The model under review builds one solid part; all positions refer to its coordinate system, in mm. Face numbers are marked on the shaded views. A direction names the side the tool comes from. Coordinates: 2 decimals unless noted, no trailing zeros. Loops run counter-clockwise (first coordinate to the right, second up) from the corner with the lowest first, then second, coordinate; pieces in that order, holes last. Notation, with made-up numbers: M 0,38 L 44,38 A18 cw 44,67 Z; hole C 75,-8 d7. An arc over 180 degrees is marked long. Use one line per item in the form item = value.
```python
from build123d import *

# Parameters (mm, degrees)
SKETCH_2_R           = 38.25
SKETCH_2_R_2         = 1.3
EXTRUDE_1_DEPTH      = 27
EXTRUDE_2_DEPTH      = 6.2
SKETCH_4_R           = 19.25
CUT_EXTRUDE_1_DEPTH  = 1.7
SKETCH_5_R           = 14.9
CUT_EXTRUDE_2_DEPTH  = 3.2
SKETCH_6_R           = 1.5
CUT_EXTRUDE_3_DEPTH  = 8
SKETCH_7_R           = 2
CUT_EXTRUDE_4_DEPTH  = 4.5
SKETCH_8_R           = 32.3
EXTRUDE_3_DEPTH      = 39.3
FILLET_1_R           = 7
FILLET_2_R           = 10
SKETCH_9_W           = 22
SKETCH_9_H           = 6
CUT_EXTRUDE_5_DEPTH  = 15
SKETCH_10_W          = 22
SKETCH_10_H          = 13
CUT_EXTRUDE_6_DEPTH  = 15
SKETCH_12_R          = 9.8
CUT_EXTRUDE_7_DEPTH  = 6.5
SKETCH_13_R          = 4
CUT_EXTRUDE_8_DEPTH  = 6
SKETCH_14_R          = 2.7
CUT_EXTRUDE_9_DEPTH  = 7
SKETCH_15_R          = 1.2
CUT_EXTRUDE_10_DEPTH = 4
SKETCH_16_R          = 1.3
SKETCH_16_R_2        = 1.2
EXTRUDE_4_DEPTH      = 12
SKETCH_18_R          = 1.3
EXTRUDE_5_DEPTH      = 9
SKETCH_19_R          = 1.5
CUT_EXTRUDE_11_DEPTH = 10


with BuildPart() as part:
    # 草图2 → 凸台-拉伸1 (new body)
    with BuildSketch(Plane(origin=(0, 0, 0), x_dir=(1, 0, 0), z_dir=(0, 1, 0))):
        with Locations(Location((0, 0, 0), (0, 0, 270))):
            Circle(SKETCH_2_R)
        with Locations(Location((0, 34.5, 0), (0, 0, 270))):
            Circle(SKETCH_2_R_2, mode=Mode.SUBTRACT)
        with Locations(Location((-24.395183951, 24.395183951, 0), (0, 0, 270))):
            Circle(SKETCH_2_R_2, mode=Mode.SUBTRACT)
        with Locations(Location((-34.5, 0, 0), (0, 0, 270))):
            Circle(SKETCH_2_R_2, mode=Mode.SUBTRACT)
        with Locations(Location((-24.395183951, -24.395183951, 0), (0, 0, 270))):
            Circle(SKETCH_2_R_2, mode=Mode.SUBTRACT)
        with Locations(Location((0, -34.5, 0), (0, 0, 270))):
            Circle(SKETCH_2_R_2, mode=Mode.SUBTRACT)
        with Locations(Location((24.395183951, -24.395183951, 0), (0, 0, 270))):
            Circle(SKETCH_2_R_2, mode=Mode.SUBTRACT)
        with Locations(Location((34.5, 0, 0), (0, 0, 270))):
            Circle(SKETCH_2_R_2, mode=Mode.SUBTRACT)
        with Locations(Location((24.395183951, 24.395183951, 0), (0, 0, 270))):
            Circle(SKETCH_2_R_2, mode=Mode.SUBTRACT)
    extrude(amount=EXTRUDE_1_DEPTH)

    # 草图3 → 凸台-拉伸2 (add)
    with BuildSketch(Plane(origin=(0, 27, 0), x_dir=(1, 0, 0), z_dir=(0, 1, 0))):
        with BuildLine():
            Line((-13.978197309, 23.1), (13.978197309, 23.1))
            ThreePointArc((13.978197309, 23.1), (27, 0), (13.978197309, -23.1))
            Line((13.978197309, -23.1), (-13.978197309, -23.1))
            ThreePointArc((-13.978197309, -23.1), (-27, 0), (-13.978197309, 23.1))
        make_face()
    extrude(amount=EXTRUDE_2_DEPTH)

    # 草图4 → 切除-拉伸1 (cut)
    with BuildSketch(Plane(origin=(0, 33.2, 0), x_dir=(1, 0, 0), z_dir=(0, 1, 0))):
        with Locations(Location((0, 0, 0), (0, 0, 270))):
            Circle(SKETCH_4_R)
    extrude(amount=-CUT_EXTRUDE_1_DEPTH, mode=Mode.SUBTRACT)

    # 草图5 → 切除-拉伸2 (cut)
    with BuildSketch(Plane(origin=(0, 33.2, 0), x_dir=(1, 0, 0), z_dir=(0, 1, 0))):
        with Locations(Location((0, 0, 0), (0, 0, 270))):
            Circle(SKETCH_5_R)
    extrude(amount=-CUT_EXTRUDE_2_DEPTH, mode=Mode.SUBTRACT)

    # 草图6 → 切除-拉伸3 (cut)
    with BuildSketch(Plane(origin=(0, 30, 0), x_dir=(1, 0, 0), z_dir=(0, 1, 0))):
        with Locations(Location((0, -12.5, 0), (0, 0, 270))):
            Circle(SKETCH_6_R)
        with Locations(Location((10.825317547, -6.25, 0), (0, 0, 270))):
            Circle(SKETCH_6_R)
        with Locations(Location((10.825317547, 6.25, 0), (0, 0, 270))):
            Circle(SKETCH_6_R)
        with Locations(Location((-10.825317547, -6.25, 0), (0, 0, 270))):
            Circle(SKETCH_6_R)
        with Locations(Location((-10.825317547, 6.25, 0), (0, 0, 270))):
            Circle(SKETCH_6_R)
        with Locations(Location((0, 12.5, 0), (0, 0, 270))):
            Circle(SKETCH_6_R)
    extrude(amount=-CUT_EXTRUDE_3_DEPTH, mode=Mode.SUBTRACT)

    # 草图7 → 切除-拉伸4 (cut)
    with BuildSketch(Plane(origin=(0, 30, 0), x_dir=(1, 0, 0), z_dir=(0, 1, 0))):
        with Locations(Location((-12.5, 0, 0), (0, 0, 270))):
            Circle(SKETCH_7_R)
        with Locations(Location((6.25, -10.825317547, 0), (0, 0, 270))):
            Circle(SKETCH_7_R)
        with Locations(Location((6.25, 10.825317547, 0), (0, 0, 270))):
            Circle(SKETCH_7_R)
    extrude(amount=-CUT_EXTRUDE_4_DEPTH, mode=Mode.SUBTRACT)

    # 草图8 → 凸台-拉伸3 (add)
    with BuildSketch(Plane(origin=(0, 0, 0), x_dir=(1, 0, 0), z_dir=(0, 1, 0))):
        with Locations(Location((0, 0, 0), (0, 0, 270))):
            Circle(SKETCH_8_R)
    extrude(amount=-EXTRUDE_3_DEPTH)

    # 圆角1
    fillet_1_edges = [part.edges().sort_by_distance(p)[0] for p in [
        (0, -39.3, -32.3),
    ]]
    fillet(fillet_1_edges, radius=FILLET_1_R)

    # 圆角2
    fillet_2_edges = [part.edges().sort_by_distance(p)[0] for p in [
        (-13.978197309, 30.1, -23.1),
        (-13.978197309, 30.1, 23.1),
        (13.978197309, 30.1, 23.1),
        (13.978197309, 30.1, -23.1),
    ]]
    fillet(fillet_2_edges, radius=FILLET_2_R)

    # 草图9 → 切除-拉伸5 (cut)
    with BuildSketch(Plane.XY.offset(40)):
        with Locations((0, -29.3)):
            Rectangle(SKETCH_9_W, SKETCH_9_H)
    extrude(amount=-CUT_EXTRUDE_5_DEPTH, mode=Mode.SUBTRACT)

    # 草图10 → 切除-拉伸6 (cut)
    with BuildSketch(Plane.XY.offset(-40)):
        with Locations((0, -30.8)):
            Rectangle(SKETCH_10_W, SKETCH_10_H)
    extrude(amount=CUT_EXTRUDE_6_DEPTH, mode=Mode.SUBTRACT)

    # 草图12 → 切除-拉伸7 (cut)
    with BuildSketch(Plane(origin=(0, 30, 0), x_dir=(1, 0, 0), z_dir=(0, 1, 0))):
        with Locations(Location((0, 0, 0), (0, 0, 270))):
            Circle(SKETCH_12_R)
    extrude(amount=-CUT_EXTRUDE_7_DEPTH, mode=Mode.SUBTRACT)

    # 草图13 → 切除-拉伸8 (cut)
    with BuildSketch(Plane(origin=(0, 23.5, 0), x_dir=(1, 0, 0), z_dir=(0, 1, 0))):
        with Locations(Location((0, 0, 0), (0, 0, 270))):
            Circle(SKETCH_13_R)
    extrude(amount=-CUT_EXTRUDE_8_DEPTH, mode=Mode.SUBTRACT)

    # 草图14 → 切除-拉伸9 (cut)
    with BuildSketch(Plane(origin=(0, 27, 0), x_dir=(1, 0, 0), z_dir=(0, 1, 0))):
        with Locations(Location((31.873843872, 13.202578417, 0), (0, 0, 270))):
            Circle(SKETCH_14_R)
        with Locations(Location((31.873843872, -13.202578417, 0), (0, 0, 270))):
            Circle(SKETCH_14_R)
        with Locations(Location((13.202578417, -31.873843872, 0), (0, 0, 270))):
            Circle(SKETCH_14_R)
        with Locations(Location((-13.202578417, -31.873843872, 0), (0, 0, 270))):
            Circle(SKETCH_14_R)
        with Locations(Location((-31.873843872, -13.202578417, 0), (0, 0, 270))):
            Circle(SKETCH_14_R)
        with Locations(Location((-31.873843872, 13.202578417, 0), (0, 0, 270))):
            Circle(SKETCH_14_R)
        with Locations(Location((-13.202578417, 31.873843872, 0), (0, 0, 270))):
            Circle(SKETCH_14_R)
        with Locations(Location((13.202578417, 31.873843872, 0), (0, 0, 270))):
            Circle(SKETCH_14_R)
    extrude(amount=-CUT_EXTRUDE_9_DEPTH, mode=Mode.SUBTRACT)

    # 草图15 → 切除-拉伸10 (cut)
    with BuildSketch(Plane.XZ):
        with Locations(Location((13.202578417, 31.873843872, 0), (0, 0, 270))):
            Circle(SKETCH_15_R)
        with Locations(Location((-13.202578417, 31.873843872, 0), (0, 0, 270))):
            Circle(SKETCH_15_R)
        with Locations(Location((-31.873843872, 13.202578417, 0), (0, 0, 270))):
            Circle(SKETCH_15_R)
        with Locations(Location((-31.873843872, -13.202578417, 0), (0, 0, 270))):
            Circle(SKETCH_15_R)
        with Locations(Location((-13.202578417, -31.873843872, 0), (0, 0, 270))):
            Circle(SKETCH_15_R)
        with Locations(Location((13.202578417, -31.873843872, 0), (0, 0, 270))):
            Circle(SKETCH_15_R)
        with Locations(Location((31.873843872, -13.202578417, 0), (0, 0, 270))):
            Circle(SKETCH_15_R)
        with Locations(Location((31.873843872, 13.202578417, 0), (0, 0, 270))):
            Circle(SKETCH_15_R)
    extrude(amount=-CUT_EXTRUDE_10_DEPTH, mode=Mode.SUBTRACT)

    # 草图16 → 凸台-拉伸4 (add)
    # profile 1 of 6: a face of its own
    with BuildSketch(Plane.XZ):
        with Locations(Location((-24.395183951, -24.395183951, 0), (0, 0, 270))):
            Circle(SKETCH_16_R)
    # profile 2 of 6: a face of its own
    with BuildSketch(Plane.XZ):
        with Locations(Location((0, -34.5, 0), (0, 0, 270))):
            Circle(SKETCH_16_R)
        with Locations(Location((0, -34.5, 0), (0, 0, 270))):
            Circle(SKETCH_16_R_2, mode=Mode.SUBTRACT)
    # profile 3 of 6: a face of its own
    with BuildSketch(Plane.XZ):
        with Locations(Location((24.395183951, -24.395183951, 0), (0, 0, 270))):
            Circle(SKETCH_16_R)
    # profile 4 of 6: a face of its own
    with BuildSketch(Plane.XZ):
        with Locations(Location((24.395183951, 24.395183951, 0), (0, 0, 270))):
            Circle(SKETCH_16_R)
    # profile 5 of 6: a face of its own
    with BuildSketch(Plane.XZ):
        with Locations(Location((0, 34.5, 0), (0, 0, 270))):
            Circle(SKETCH_16_R)
        with Locations(Location((0, 34.5, 0), (0, 0, 270))):
            Circle(SKETCH_16_R_2, mode=Mode.SUBTRACT)
    # profile 6 of 6: a face of its own
    with BuildSketch(Plane.XZ):
        with Locations(Location((-24.395183951, 24.395183951, 0), (0, 0, 270))):
            Circle(SKETCH_16_R)
    extrude(amount=-EXTRUDE_4_DEPTH)

    # 草图18 → 凸台-拉伸5 (add)
    with BuildSketch(Plane(origin=(0, 8, 0), x_dir=(-1, 0, 0), z_dir=(0, -1, 0))):
        with Locations(Location((34.5, 0, 0), (0, 0, 90))):
            Circle(SKETCH_18_R)
        with Locations(Location((-34.5, 0, 0), (0, 0, 90))):
            Circle(SKETCH_18_R)
    extrude(amount=-EXTRUDE_5_DEPTH)

    # 草图19 → 切除-拉伸11 (cut)
    with BuildSketch(Plane(origin=(0, 27, 0), x_dir=(1, 0, 0), z_dir=(0, 1, 0))):
        with Locations(Location((-34.5, 0, 0), (0, 0, 270))):
            Circle(SKETCH_19_R)
        with Locations(Location((34.5, 0, 0), (0, 0, 270))):
            Circle(SKETCH_19_R)
    extrude(amount=-CUT_EXTRUDE_11_DEPTH, mode=Mode.SUBTRACT)


solid = part.part
```
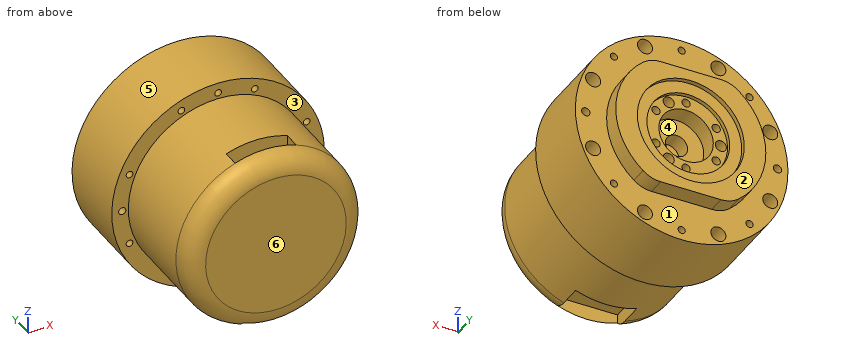
1. Machinability: for the marked faces 1, 2 and 3, which of the approach directions +Z, -Z, +X, -X, +Y, -Y give a long, thin tool a straight path to every point of the face, cutting with its end or side? Answer none if there is none.
Response values:
face_1 = +Y
face_2 = +Z, -Z, +X, -X, +Y
face_3 = -Y
2. Add section C-C (y = -2). State the section outline as (x, z) points, then the cut area to 3 significant figures.
Response values:
outline = C 0,0 d64.6
area = 3,280 mm^2
3. Insertion check: P1, Ø1.6, axis at x = 24.4, z = 24.4, coming from the -Y side; P2, Ø3, axis at x = 26, z = -21.5, coming from the +Y side; P3, Ø1.5, axis at x = -3.5, y = -4.5, coming from the +Z side. Each pin has a flat end and moves straight along its axis. Give the tip position at first contact, or say it passes through.
Response values:
P1 = 0
P2 = 27
P3 = 32.18
4. Add section B-B (x = 0). Count the separate pieces of the cut face and the enclosed holes in it, then the cut area to 3 significant figures.
Response values:
separate_pieces = 3
enclosed_holes = 0
area = 4,270 mm^2
5. The part is to be moulded in two halves that separate along Z. For the marked faces 4, 5 and 6, say which applies: pulls with the +Z half, pulls with the -Z half, needs draft (parallel to the pull), parting line crosses it, or undercut.
Response values:
face_4 = undercut
face_5 = parting line crosses it
face_6 = needs draft
6. Add section A-A (y = 10.5). State the section outline as (x, z) points.
Response values:
outline = C 0,0 d76.5; hole C 0,-34.5 d2.4; hole C 0,34.5 d2.4
7. Wall thickness on line 1 along X through (y, z) = (20, 0); line 2 along Z through (x, y) = (-32, 21.5); line 3 along X through (y, z) = (19.5, 1): over which ranges is each line inside the solid? List them lowest first. Write a range as from..to.
Response values:
line_1 = -38.25..-36, -33..-4, 4..33, 36..38.25
line_2 = -20.95..-15.9, -10.51..10.51, 15.9..20.95
line_3 = -38.24..-35.62, -33.38..-3.87, 3.87..33.38, 35.62..38.24
